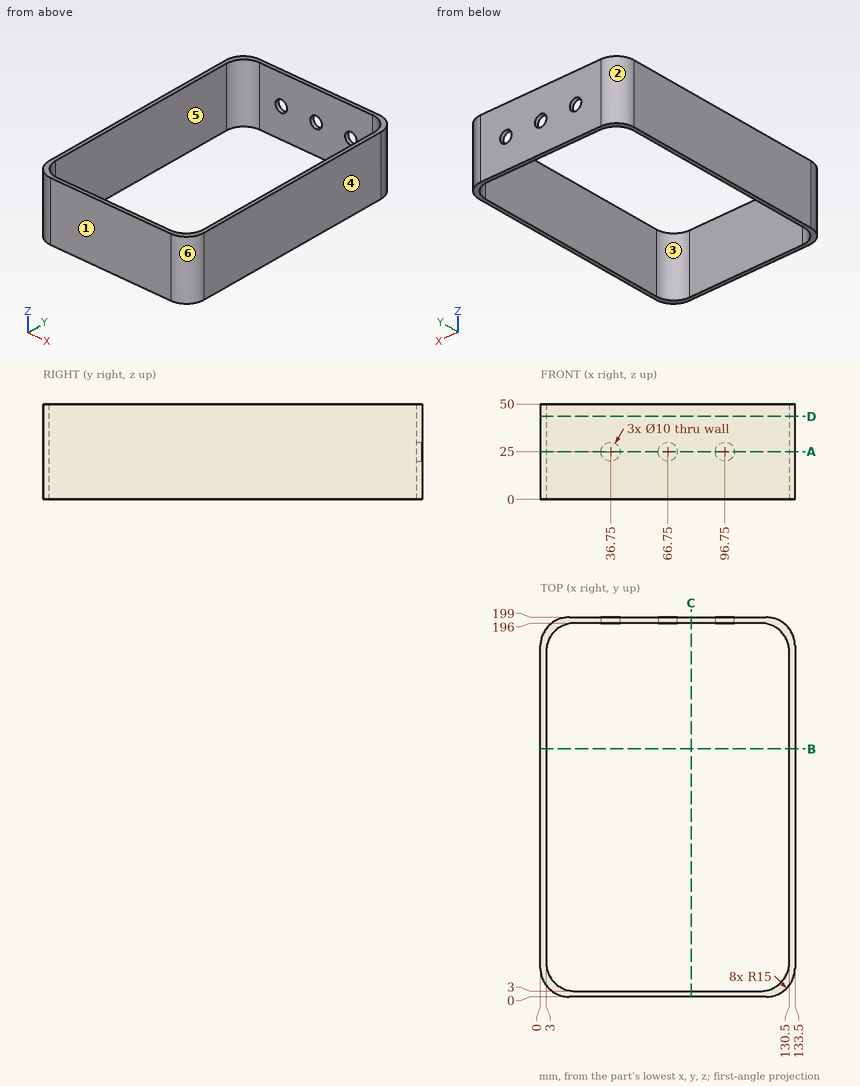
Here's the drawing with two shaded views (mm, measured from the low corner). I have some questions. A direction names the side the tool comes from. Round coordinates to 2 decimals unless told otherwise and drop trailing zeros. Loops run counter-clockwise (first coordinate to the right, second up) from the corner with the lowest first, then second, coordinate; pieces in that order, holes last.
Item 1: Suppose I cut it at D-D, the plane z = 43.5. Write out the boundary of the cut face in (x, y).
Item 2: Suppose I cut it at A-A, the plane z = 25. Write out the boundary of the cut face in (x, y).
Item 3: Which directions (+Z, -Z, +X, -X, +Y, -Y) give clear straight access to the entire face, cutting with the end or side of a thin tool? Please do the marked faces 5 and 6.
Item 4: Suppose I cut it at C-C, the plane x = 79. Write out the boundary of the cut face in (y, z).
Item 5: Please list where these lines run through material, in increasing order: L1, parallel to Z at x = 96.75, y = 198.15; L2, parallel to Y at x = 20, z = 38.5; L3, parallel to X at y = 153, z = 18.
Item 6: If we mould it in two halves opening along X, with no side actions, what happens to the marked faces 1, 2, 3 and 4? For each: +X half, -X half, draft (parallel to the pull), parting line (faces both ways), or undercut.
Item 7: Suppose I cut it at B-B, the plane y = 130. Write out the boundary of the cut face in (x, z), then the cut area to 3 significant figures.
Reported:
1. outline: (0, 15) arc R15 ccw to (15, 0) - (118.5, 0) arc R15 ccw to (133.5, 15) - (133.5, 184) arc R15 ccw to (118.5, 199) - (15, 199) arc R15 ccw to (0, 184) - close; hole (3, 18) arc R15 ccw to (18, 3) - (115.5, 3) arc R15 ccw to (130.5, 18) - (130.5, 181) arc R15 ccw to (115.5, 196) - (18, 196) arc R15 ccw to (3, 181) - close
2. outline: (0, 15) arc R15 ccw to (15, 0) - (118.5, 0) arc R15 ccw to (133.5, 15) - (133.5, 184) arc R15 ccw to (118.5, 199) - (101.75, 199) - (101.75, 196) - (115.5, 196) arc R15 cw to (130.5, 181) - (130.5, 18) arc R15 cw to (115.5, 3) - (18, 3) arc R15 cw to (3, 18) - (3, 181) arc R15 cw to (18, 196) - (31.75, 196) - (31.75, 199) - (15, 199) arc R15 ccw to (0, 184) - close; (41.75, 196) - (61.75, 196) - (61.75, 199) - (41.75, 199) - close; (71.75, 196) - (91.75, 196) - (91.75, 199) - (71.75, 199) - close
3. face 5: +Z, -Z
3. face 6: +Z, -Z, +X, -Y
4. outline: (0, 0) - (3, 0) - (3, 50) - (0, 50) - close; (196, 0) - (199, 0) - (199, 50) - (196, 50) - close
5. L1: z = 0 to 20, 30 to 50
5. L2: y = 0 to 3, 196 to 199
5. L3: x = 0 to 3, 130.5 to 133.5
6. face 1: draft
6. face 2: -X half
6. face 3: undercut
6. face 4: +X half
7. outline: (0, 0) - (3, 0) - (3, 50) - (0, 50) - close; (130.5, 0) - (133.5, 0) - (133.5, 50) - (130.5, 50) - close
7. area: 300 mm2
